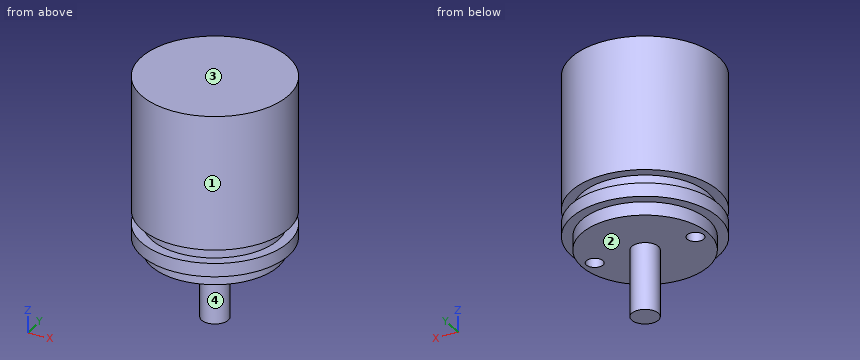
from build123d import *

# Parameters (mm, degrees)
SKETCH1_R           = 2
BOSS_EXTRUDE1_DEPTH = 10
SKETCH2_R           = 9.5
BOSS_EXTRUDE2_DEPTH = 2
SKETCH3_R           = 11
BOSS_EXTRUDE3_DEPTH = 2
SKETCH4_R           = 9.5
BOSS_EXTRUDE4_DEPTH = 2
SKETCH5_R           = 11
BOSS_EXTRUDE5_DEPTH = 20
SKETCH6_R           = 1.25
CUT_EXTRUDE1_DEPTH  = 5


with BuildPart() as part:
    # Sketch1 → Boss-Extrude1 (new body)
    with BuildSketch(Plane.XY):
        Circle(SKETCH1_R)
    extrude(amount=BOSS_EXTRUDE1_DEPTH)

    # Sketch2 → Boss-Extrude2 (add)
    with BuildSketch(Plane.XY.offset(10)):
        Circle(SKETCH2_R)
    extrude(amount=BOSS_EXTRUDE2_DEPTH)

    # Sketch3 → Boss-Extrude3 (add)
    with BuildSketch(Plane.XY.offset(12)):
        Circle(SKETCH3_R)
    extrude(amount=BOSS_EXTRUDE3_DEPTH)

    # Sketch4 → Boss-Extrude4 (add)
    with BuildSketch(Plane.XY.offset(14)):
        Circle(SKETCH4_R)
    extrude(amount=BOSS_EXTRUDE4_DEPTH)

    # Sketch5 → Boss-Extrude5 (add)
    with BuildSketch(Plane.XY.offset(16)):
        Circle(SKETCH5_R)
    extrude(amount=BOSS_EXTRUDE5_DEPTH)

    # Sketch6 → Cut-Extrude1 (cut)
    with BuildSketch(Plane(origin=(0, 0, 10), x_dir=(-1, 0, 0), z_dir=(0, 0, -1))):
        with Locations((-7.5, 0)):
            Circle(SKETCH6_R)
        with Locations((7.5, 0)):
            Circle(SKETCH6_R)
    extrude(amount=-CUT_EXTRUDE1_DEPTH, mode=Mode.SUBTRACT)


solid = part.part
Source: CAD feature listing. Evaluate the final solid. Frame: model axes, mm. Face numbers are marked on the shaded views. A direction names the side the tool comes from. Give positions to 0.01 mm unless a question says otherwise; leave off trailing zeros. Write each loop counter-clockwise with the first axis right and the second up, starting at its lowest first coordinate (ties: lowest second). Pieces come first, ordered by that corner, then holes. Notation, with made-up numbers: M 67.25,76 L 117.25,76 A20 ccw 117.25,109 Z; hole C 46,-4.75 d9. An arc over 180 degrees is marked long. Answer as a JSON object with one key per item and string values.
Q1. Access query for the marked faces 3 and 4. Directions: +Z, -Z, +X, -X, +Y, -Y. A direction counts if a zero-diameter tool reaches every point of the face in a straight line with its end or side. Return the directions, or none.
Geometry check:
{"face 3": "+Z, +X, -X, +Y, -Y", "face 4": "-Z"}
Q2. Ray query, line 1 along Z through (x, y) = (-5.5, -9.25); line 2 along Z through (x, y) = (-6.25, -3); line 3 along Y through (x, z) = (-7.5, 11.8). Return the intervals inside material, ascending.
Geometry check:
{"line 1": "z = 12 to 14, 16 to 36", "line 2": "z = 10 to 36", "line 3": "y = -5.83 to -1.25, 1.25 to 5.83"}
Q3. Cut plane C-C, the plane z = 11. Return the cut outline in (x, y), then the cut area to 3 significant figures.
Geometry check:
{"outline": "C 0,0 d19; hole C -7.5,0 d2.5; hole C 7.5,0 d2.5", "area": "274 mm^2"}
Q4. Cut plane D-D, the plane z = 18. Return the cut outline in (x, y), then the cut area to 3 significant figures.
Geometry check:
{"outline": "C 0,0 d22", "area": "380 mm^2"}
Q5. Mould query, pull axis X, two halves, no side actions, for the marked faces 1 and 2. Classes: +X half, -X half, draft (parallel to the pull), parting line (faces both ways), or undercut.
Geometry check:
{"face 1": "parting line", "face 2": "draft"}
Q6. Contact query for flat-ended pins moving along their axis: P1, Ø2, axis at y = 7.5, z = 13, coming from the +X side; P2, Ø3, axis at x = -7, y = 0, coming from the -Z side; P3, Ø4, axis at y = 0, z = 11, coming from the +X side; P4, Ø3, axis at x = -3, z = 6.5, coming from the -Y side. Output: stop coordinate, or through.
Geometry check:
{"P1": "stops at x = 8.87", "P2": "stops at z = 10", "P3": "stops at x = 11", "P4": "stops at y = -1.32"}
Q7. Cut plane A-A, the plane x = 0. Return the cut outline in (y, z), then the cut area to 3 significant figures.
Geometry check:
{"outline": "M -11,12 L -9.5,12 L -9.5,10 L -2,10 L -2,0 L 2,0 L 2,10 L 9.5,10 L 9.5,12 L 11,12 L 11,14 L 9.5,14 L 9.5,16 L 11,16 L 11,36 L -11,36 L -11,16 L -9.5,16 L -9.5,14 L -11,14 Z", "area": "600 mm^2"}
Q8. Cut plane B-B, the plane y = 0. Return the cut outline in (x, z), then the cut area to 3 significant figures.
Geometry check:
{"outline": "M -11,12 L -9.5,12 L -9.5,10 L -8.75,10 L -8.75,15 L -6.25,15 L -6.25,10 L -2,10 L -2,0 L 2,0 L 2,10 L 6.25,10 L 6.25,15 L 8.75,15 L 8.75,10 L 9.5,10 L 9.5,12 L 11,12 L 11,14 L 9.5,14 L 9.5,16 L 11,16 L 11,36 L -11,36 L -11,16 L -9.5,16 L -9.5,14 L -11,14 Z", "area": "575 mm^2"}
